Geometry: final body of the model. Coordinates: model frame, mm. Coordinates: 2 decimals unless noted, no trailing zeros. Write each loop counter-clockwise with the first axis right and the second up, starting at its lowest first coordinate (ties: lowest second). Pieces come first, ordered by that corner, then holes. Notation, with made-up numbers: (-8.5, -7.75) - (16.5, -7.75) arc R34 cw to (16.5, 26.25) - close; hole circle Ø5 at (-19.5, -34). An arc over 180 degrees is marked (long way). Answer as a JSON object with one key per item and string values. Group by question number.
Item 1: Section A-A on z = 0.6. State how many separate pieces and enclosed holes the cut face has, and give its area (3 significant figures).
Item 2: Mould query, pull axis Y, two halves, no side actions, for faces 1 (the cylindrical face through (-9.391, 23.614, 1.479)), 2 (the flat face through (-16, 27, 0)), 3 (the cylindrical face through (5.653, 26.614, 1.479)), 4 (the cylindrical face through (-20.402, 23.912, 1.479)). Classes: pulls with the +Y half, pulls with the -Y half, needs draft (parallel to the pull), parting line crosses it, or undercut.
Item 3: Section B-B on y = 21.25. Return loops of the section in (x, z), and give its area (3 significant figures).
Item 4: Line query: line 1 along Y through (x, z) = (-16, 1.65); line 2 along X through (y, z) = (23.5, 2.7); line 3 along X through (y, z) = (25, 0.85). Output: solid intervals per line, ascending. Write a range as from..to.
```python
from build123d import *

# Parameters (mm, degrees)
SKETCH1_W                = 68.327661803
SKETCH1_H                = 52.686389824
BOSS_EXTRUDE1_DEPTH      = 3
CUT_EXTRUDE1_DEPTH       = 100
SKETCH4_W                = 3
SKETCH4_H                = 16.961263462
BOSS_EXTRUDE2_DEPTH      = 4
SKETCH5_W                = 3
SKETCH5_H                = 16.961263462
BOSS_EXTRUDE3_DEPTH      = 39.5
SKETCH6_W                = 3
SKETCH6_H                = 16.961263462
BOSS_EXTRUDE4_DEPTH      = 35.754290268
FILLET1_R                = 7.5
FILLET2_R                = 7.5
FILLET3_R                = 7.5
FILLET4_R                = 7.5
SKETCH9_R                = 0.5
CUT_EXTRUDE5_DEPTH       = 14
SKETCH7_R                = 0.5
CUT_EXTRUDE6_DEPTH       = 14
SKETCH10_R               = 2.35
CUT_EXTRUDE7_DEPTH       = 10
SKETCH11_R               = 2.35
CUT_EXTRUDE8_DEPTH       = 10
SKETCH12_R               = 1.5
CUT_EXTRUDE9_DEPTH       = 10
CUT_EXTRUDE_4_DEPTH      = 63.27060323
CUT_EXTRUDE_4_DEPTH_BACK = 63.27060323
SKETCH_2_W               = 38.540786773
SKETCH_2_H               = 30.686503212
SKETCH_1_W               = 58.401406077
SKETCH_1_H               = 28.148942287
SKETCH_1_R               = 0.5
SKETCH_1_W_2             = 30
SKETCH_1_H_2             = 7
SKETCH_1_R_2             = 1.75
CUT_EXTRUDE_7_DEPTH      = 51.962343493
SKETCH_3_W               = 7.5
SKETCH_3_H               = 7
SKETCH_3_R               = 1.75
EXTRUDE_1_DEPTH          = 3
FILLET_2_R               = 3.5


with BuildPart() as part:
    # Sketch1 → Boss-Extrude1 (new body)
    with BuildSketch(Plane.XY):
        with Locations((-34.163830901, 26.343194912)):
            Rectangle(SKETCH1_W, SKETCH1_H)
    extrude(amount=BOSS_EXTRUDE1_DEPTH)

    # Sketch2 → Cut-Extrude1 (cut)
    with BuildSketch(Plane(origin=(0, 0, 0), x_dir=(-1, 0, 0), z_dir=(0, 0, -1))):
        Polygon((34.754290268, 32.233658713), (0, 32.233658713), (0, 52.686389824), (34.754290268, 52.686389824), (68.327661803, 52.686389824), (68.327661803, 0), (34.754290268, 0), (0, 0), (0, 15.272395251), (34.754290268, 15.272395251), align=None)
    extrude(amount=-CUT_EXTRUDE1_DEPTH, mode=Mode.SUBTRACT)

    # Sketch4 → Boss-Extrude2 (add)
    with BuildSketch(Plane.ZY.offset(34.754290268)):
        with Locations((1.5, 23.753026982)):
            Rectangle(SKETCH4_W, SKETCH4_H)
    extrude(amount=BOSS_EXTRUDE2_DEPTH)

    # Sketch5 → Boss-Extrude3 (add)
    with BuildSketch(Plane(origin=(0, 0, 0), x_dir=(-1, 0, 0), z_dir=(0, 0, -1))):
        with Locations((37.254290268, 23.753026982)):
            Rectangle(SKETCH5_W, SKETCH5_H)
    extrude(amount=BOSS_EXTRUDE3_DEPTH)

    # Sketch6 → Boss-Extrude4 (add)
    with BuildSketch(Plane(origin=(-35.754290268, 0, 0), x_dir=(0, 0, -1), z_dir=(1, 0, 0))):
        with Locations((38, 23.753026982)):
            Rectangle(SKETCH6_W, SKETCH6_H)
    extrude(amount=BOSS_EXTRUDE4_DEPTH)

    # Fillet1
    fillet1_edges = [part.edges().sort_by_distance(p)[0] for p in [
        (0, 15.272395251, 1.5),
    ]]
    fillet(fillet1_edges, radius=FILLET1_R)

    # Fillet2
    fillet2_edges = [part.edges().sort_by_distance(p)[0] for p in [
        (0, 32.233658713, 1.5),
    ]]
    fillet(fillet2_edges, radius=FILLET2_R)

    # Fillet3
    fillet3_edges = [part.edges().sort_by_distance(p)[0] for p in [
        (0, 32.233658713, -38),
    ]]
    fillet(fillet3_edges, radius=FILLET3_R)

    # Fillet4
    fillet4_edges = [part.edges().sort_by_distance(p)[0] for p in [
        (0, 15.272395251, -38),
    ]]
    fillet(fillet4_edges, radius=FILLET4_R)

    # Sketch9 → Cut-Extrude5 (cut)
    with BuildSketch(Plane.ZY.offset(38.754290268)):
        with Locations((-13.849226824, 24.283657668)):
            Circle(SKETCH9_R)
        with Locations((-11.849226824, 24.283657668)):
            Circle(SKETCH9_R)
        with Locations((-18.799226824, 19.683657668)):
            Circle(SKETCH9_R)
        with Locations((-18.799226824, 17.683657668)):
            Circle(SKETCH9_R)
        with Locations((-23.149226824, 24.283657668)):
            Circle(SKETCH9_R)
        with Locations((-25.149226824, 24.283657668)):
            Circle(SKETCH9_R)
        with Locations((-18.799226824, 30.633657668)):
            Circle(SKETCH9_R)
        with Locations((-18.799226824, 28.633657668)):
            Circle(SKETCH9_R)
    extrude(amount=-CUT_EXTRUDE5_DEPTH, mode=Mode.SUBTRACT)

    # Sketch7 → Cut-Extrude6 (cut)
    with BuildSketch(Plane(origin=(0, 0, 0), x_dir=(-1, 0, 0), z_dir=(0, 0, -1))):
        with Locations((15.785473329, 30.515840692)):
            Circle(SKETCH7_R)
        with Locations((15.805568543, 28.515941649)):
            Circle(SKETCH7_R)
        with Locations((20.799025765, 24.215896885)):
            Circle(SKETCH7_R)
        with Locations((22.798924808, 24.235992099)):
            Circle(SKETCH7_R)
        with Locations((11.499495215, 24.12245414)):
            Circle(SKETCH7_R)
        with Locations((9.499596172, 24.102358926)):
            Circle(SKETCH7_R)
        with Locations((15.895494626, 19.566393431)):
            Circle(SKETCH7_R)
        with Locations((15.91558984, 17.566494388)):
            Circle(SKETCH7_R)
    extrude(amount=-CUT_EXTRUDE6_DEPTH, mode=Mode.SUBTRACT)

    # Sketch10 → Cut-Extrude7 (cut)
    with BuildSketch(Plane.ZY.offset(38.754290268)):
        with Locations((-18.799226824, 24.283657668)):
            Circle(SKETCH10_R)
    extrude(amount=-CUT_EXTRUDE7_DEPTH, mode=Mode.SUBTRACT)

    # Sketch11 → Cut-Extrude8 (cut)
    with BuildSketch(Plane(origin=(0, 0, 0), x_dir=(-1, 0, 0), z_dir=(0, 0, -1))):
        with Locations((15.849275634, 24.16616123)):
            Circle(SKETCH11_R)
    extrude(amount=-CUT_EXTRUDE8_DEPTH, mode=Mode.SUBTRACT)

    # Sketch12 → Cut-Extrude9 (cut)
    with BuildSketch(Plane.XY.offset(-36.5)):
        with Locations((-15.849275634, 24.16616123)):
            Circle(SKETCH12_R)
    extrude(amount=-CUT_EXTRUDE9_DEPTH, mode=Mode.SUBTRACT)

    # 草圖2 → 除料-伸長4 (cut, two sides: drawn at the far end of the back side and taken through both)
    with BuildSketch(Plane(origin=(-35.754290268, 0, 0), x_dir=(0, 0, -1), z_dir=(1, 0, 0)).offset(-CUT_EXTRUDE_4_DEPTH_BACK)):
        with Locations((23.770839113, 24.432880731)):
            Rectangle(SKETCH_2_W, SKETCH_2_H)
    extrude(amount=CUT_EXTRUDE_4_DEPTH + CUT_EXTRUDE_4_DEPTH_BACK, mode=Mode.SUBTRACT)

    # 草圖1 → 除料-伸長7 (cut, through all)
    # profile 1 of 4: a face of its own
    with BuildSketch(Plane.XY.offset(3)):
        with Locations((-17.675205009, 24.250222974)):
            Rectangle(SKETCH_1_W, SKETCH_1_H)
        with BuildLine():
            Line((0, 22.772395251), (0, 24.733658713))
            ThreePointArc((0, 24.733658713), (-2.196699141, 30.036959572), (-7.5, 32.233658713))
            Line((-7.5, 32.233658713), (-38.754290268, 32.233658713))
            Line((-38.754290268, 32.233658713), (-38.754290268, 15.272395251))
            Line((-38.754290268, 15.272395251), (-7.5, 15.272395251))
            ThreePointArc((-7.5, 15.272395251), (-2.196699141, 17.469094393), (0, 22.772395251))
        make_face(mode=Mode.SUBTRACT)
    # profile 2 of 4: a face of its own
    with BuildSketch(Plane.XY.offset(3)):
        with BuildLine():
            ThreePointArc((-7.5, 15.272395251), (-2.196699141, 17.469094393), (0, 22.772395251))
            Line((0, 22.772395251), (0, 24.733658713))
            ThreePointArc((0, 24.733658713), (-2.196699141, 30.036959572), (-7.5, 32.233658713))
            Line((-7.5, 32.233658713), (-38.754290268, 32.233658713))
            Line((-38.754290268, 32.233658713), (-38.754290268, 15.272395251))
            Line((-38.754290268, 15.272395251), (-7.5, 15.272395251))
        make_face()
        with Locations((-15.91558984, 17.566494388)):
            Circle(SKETCH_1_R, mode=Mode.SUBTRACT)
        with Locations((-15.805568543, 28.515941649)):
            Circle(SKETCH_1_R, mode=Mode.SUBTRACT)
        with Locations((-15.895494626, 19.566393431)):
            Circle(SKETCH_1_R, mode=Mode.SUBTRACT)
        with Locations((-15.785473329, 30.515840692)):
            Circle(SKETCH_1_R, mode=Mode.SUBTRACT)
        with Locations((-15.849275634, 24.16616123)):
            Rectangle(SKETCH_1_W_2, SKETCH_1_H_2, mode=Mode.SUBTRACT)
    # profile 3 of 4: a face of its own
    with BuildSketch(Plane.XY.offset(3)):
        with Locations((-4.849275634, 24.16616123)):
            Circle(SKETCH_1_R_2)
    # profile 4 of 4: a face of its own
    with BuildSketch(Plane.XY.offset(3)):
        with Locations((-26.849275634, 24.16616123)):
            Circle(SKETCH_1_R_2)
    extrude(amount=-CUT_EXTRUDE_7_DEPTH, mode=Mode.SUBTRACT)

    # 草圖3 → 填料-伸長1 (add, through all)
    # profile 1 of 2: a face of its own
    with BuildSketch(Plane.XY.offset(3)):
        with Locations((-34.599275634, 24.16616123)):
            Rectangle(SKETCH_3_W, SKETCH_3_H)
        with Locations((-34.849275634, 24.16616123)):
            Circle(SKETCH_3_R, mode=Mode.SUBTRACT)
    # profile 2 of 2: a face of its own
    with BuildSketch(Plane.XY.offset(3)):
        with Locations((2.900724366, 24.16616123)):
            Rectangle(SKETCH_3_W, SKETCH_3_H)
        with Locations((3.150724366, 24.16616123)):
            Circle(SKETCH_3_R, mode=Mode.SUBTRACT)
    extrude(amount=-EXTRUDE_1_DEPTH)

    # 圓角2
    fillet_2_edges = [part.edges().sort_by_distance(p)[0] for p in [
        (6.650724366, 20.66616123, 1.5),
        (6.650724366, 27.66616123, 1.5),
        (-38.349275634, 20.66616123, 1.5),
        (-38.349275634, 27.66616123, 1.5),
    ]]
    fillet(fillet_2_edges, radius=FILLET_2_R - 0.0001)  # a hair under: the kernel refuses the full size


solid = part.part
```
Checks:
{
 "1": {"separate pieces": "1", "enclosed holes": "9", "area": "246 mm^2"},
 "2": {"face 1": "undercut", "face 2": "needs draft", "face 3": "pulls with the +Y half", "face 4": "undercut"},
 "3": {"outline": "(-36.78, 0) - (5.09, 0) - (5.09, 3) - (-36.78, 3) - close", "area": "126 mm^2"},
 "4": {"line 1": "20.67..21.82, 26.51..27.67", "line 2": "-38.29..-36.47, -33.23..-28.47, -25.23..-18.1, -13.6..-6.47, -3.23..1.53, 4.77..6.59", "line 3": "-38.25..-36.39, -33.31..-28.39, -25.31..-18.05, -13.65..-6.39, -3.31..1.61, 4.69..6.55"}
}
